```python
from build123d import *

# Parameters (mm, degrees)
BOSS_EXTRUDE1_DEPTH = 2.4
SKETCH2_R           = 2.75
BOSS_EXTRUDE2_DEPTH = 3.9
FILLET1_R           = 0.7
FILLET2_R           = 0.2
M3_TAPPED_HOLE1_D   = 2.5


with BuildPart() as part:
    # Sketch1 → Boss-Extrude1 (new body)
    with BuildSketch(Plane(origin=(0, 0, 0), x_dir=(1, 0, 0), z_dir=(0, 1, 0))):
        Polygon((3.175426481, 0), (1.58771324, 2.75), (-1.58771324, 2.75), (-3.175426481, 0), (-1.58771324, -2.75), (1.58771324, -2.75), align=None)
    extrude(amount=BOSS_EXTRUDE1_DEPTH)

    # Sketch2 → Boss-Extrude2 (add)
    with BuildSketch(Plane.XZ):
        Circle(SKETCH2_R)
    extrude(amount=-BOSS_EXTRUDE2_DEPTH)

    # Fillet1
    fillet1_edges = [part.edges().sort_by_distance(p)[0] for p in [
        (-2.75, 3.9, 0),
    ]]
    fillet(fillet1_edges, radius=FILLET1_R)

    # Fillet2
    fillet2_edges = [part.edges().sort_by_distance(p)[0] for p in [
        (1.58771324, 1.2, 2.75),
        (-1.58771324, 1.2, 2.75),
        (-3.175426481, 1.2, 0),
        (-1.58771324, 1.2, -2.75),
        (1.58771324, 1.2, -2.75),
        (3.175426481, 1.2, 0),
    ]]
    fillet(fillet2_edges, radius=FILLET2_R)

    # M3 Tapped Hole1 (through all)
    with Locations(Plane(origin=(0, 0, 0), x_dir=(-1, 0, 0), z_dir=(0, -1, 0))):
        with Locations((0, 0)):
            Hole(M3_TAPPED_HOLE1_D / 2)


solid = part.part
```
Geometry: final body of the model. Coordinates: model frame, mm. A direction names the side the tool comes from. Round coordinates to 2 decimals unless told otherwise and drop trailing zeros. Loops run counter-clockwise (first coordinate to the right, second up) from the corner with the lowest first, then second, coordinate; pieces in that order, holes last. Notation, with made-up numbers: (68, -14) -> (102, -14) arc R15 ccw to (102, -10) -> close; hole circle Ø4 at (1.25, 19). An arc over 180 degrees is marked (long way). Write each question's results on one line, items separated by ' | '.
Item 1: Line query: probe 1 along Z at (x, y) = (0, 1.9); probe 2 along Z at (x, y) = (0.25, 2.8); probe 3 along X at (y, z) = (1.7, -0.55). Output: solid intervals per line, ascending. Write a range as [from, to].
Answers below:
probe 1: z = [-2.75, -1.25], [1.25, 2.75] | probe 2: z = [-2.74, -1.22], [1.22, 2.74] | probe 3: x = [-2.86, -1.12], [1.12, 2.86]
Item 2: Cut plane A-A on y = 0.4. Return the cut outline in (x, z), and give its area (3 significant figures).
Answers below:
outline: (-3.12, -0.1) -> (-1.65, -2.65) arc R0.2 ccw to (-1.47, -2.75) -> (1.47, -2.75) arc R0.2 ccw to (1.65, -2.65) -> (3.12, -0.1) arc R0.2 ccw to (3.12, 0.1) -> (1.65, 2.65) arc R0.2 ccw to (1.47, 2.75) -> (-1.47, 2.75) arc R0.2 ccw to (-1.65, 2.65) -> (-3.12, 0.1) arc R0.2 ccw to start; hole circle Ø2.5 at (0, 0) | area: 21.3 mm²
Item 3: Cut plane B-B on z = 0. Return the cut outline in (x, y), and give its area (3 significant figures).
Answers below:
outline: (-3.14, 0) -> (-1.25, 0) -> (-1.25, 3.9) -> (-2.05, 3.9) arc R0.7 ccw to (-2.75, 3.2) -> (-2.75, 2.4) -> (-3.14, 2.4) -> close; (1.25, 0) -> (3.14, 0) -> (3.14, 2.4) -> (2.75, 2.4) -> (2.75, 3.2) arc R0.7 ccw to (2.05, 3.9) -> (1.25, 3.9) -> close | area: 13.4 mm²
Item 4: Cut plane C-C on y = 3.35. Return the cut outline in (x, z), and give its area (3 significant figures).
Answers below:
outline: circle Ø5.47 at (0, 0); hole circle Ø2.5 at (0, 0) | area: 18.6 mm²
Item 5: Pin query (flat end, axial travel): pin 1 Ø0.7 at (x, z) = (-1, 2) entering from +Y; pin 2 Ø1 at (x, y) = (2.5, 2) entering from -Z; pin 3 Ø2 at (y, z) = (1, 1.5) entering from +X. Return the tip coordinate at first contact, or that it passes through.
Answers below:
pin 1: stops at y = 3.9 | pin 2: stops at z = -2.04 | pin 3: stops at x = 2.89
Item 6: Set-up query: faces 1 (the face through (1.45, 2.4, 2.52)), 2 (the face through (-1.5, 2.4, -2.5)), 3 (the face through (1.45, 2.4, -2.52)). Return all of +Z, -Z, +X, -X, +Y, -Y with unobstructed straight access to the full face (end or side cutting, diameter ignored); none if empty.
Answers below:
face 1: +Z, +X, +Y | face 2: -Z, -X, +Y | face 3: -Z, +X, +Y
